from build123d import *

# Parameters (mm, degrees)
SKETCH1_R                                   = 16
BOSS_EXTRUDE1_DEPTH                         = 7.5
SKETCH2_W                                   = 15
SKETCH2_H                                   = 17
BOSS_EXTRUDE2_DEPTH                         = 20
SKETCH3_W                                   = 70
SKETCH3_H                                   = 50
SKETCH3_R                                   = 12.5
SKETCH3_R_2                                 = 1.75
BOSS_EXTRUDE4_DEPTH                         = 15
CHAMFER1_SIZE                               = 1
CUT_EXTRUDE1_REACH                          = 72.373
SKETCH4_R                                   = 3.5
CBORE_FOR_M3_CHEESE_HEAD_SCREW3_D           = 3.4
CBORE_FOR_M3_CHEESE_HEAD_SCREW3_CBORE_D     = 6.5
CBORE_FOR_M3_CHEESE_HEAD_SCREW3_CBORE_DEPTH = 2
BOSS_EXTRUDE5_START                         = -17
BOSS_EXTRUDE5_DEPTH                         = 17
CBORE_FOR_M6_HEX_HEAD_BOLT1_AT_2_COUNT      = 2
CBORE_FOR_M6_HEX_HEAD_BOLT1_AT_2_PITCH      = 18
CBORE_FOR_M6_HEX_HEAD_BOLT1_AT_3_COUNT      = 2
CBORE_FOR_M6_HEX_HEAD_BOLT1_AT_3_PITCH      = 68.410525506
CBORE_FOR_M6_HEX_HEAD_BOLT1_AT_4_COUNT      = 2
CBORE_FOR_M6_HEX_HEAD_BOLT1_AT_4_PITCH      = 66


# Read off the part's stored shape, not the designer's step: Boss-Extrude5
with BuildPart() as part:
    # Sketch1 → Boss-Extrude1 (new, symmetric)
    with BuildSketch(Plane.XY):
        Polygon((-25, -20.805513048), (-40, -20.805513048), (-40, -3.805513048), (-25, -3.805513048), (-25, 29.194486952), (25, 29.194486952), (25, -3.805513048), (40, -3.805513048), (40, -20.805513048), (25, -20.805513048), align=None)
        with Locations((0, 4.194486952)):
            Circle(SKETCH1_R, mode=Mode.SUBTRACT)
    extrude(amount=BOSS_EXTRUDE1_DEPTH, both=True)

    # Sketch2 → Boss-Extrude2 (add)
    with BuildSketch(Plane(origin=(0, 0, -7.5), x_dir=(-1, 0, 0), z_dir=(0, 0, -1))):
        with Locations((32.5, -12.305513048)):
            Rectangle(SKETCH2_W, SKETCH2_H)
        with Locations((-32.5, -12.305513048)):
            Rectangle(SKETCH2_W, SKETCH2_H)
    extrude(amount=BOSS_EXTRUDE2_DEPTH)

    # Sketch3 → Boss-Extrude4 (add)
    with BuildSketch(Plane(origin=(0, 0, -27.5), x_dir=(-1, 0, 0), z_dir=(0, 0, -1))):
        with Locations((-5, 4.194486952)):
            Rectangle(SKETCH3_W, SKETCH3_H)
        with Locations((0, 4.194486952)):
            Circle(SKETCH3_R, mode=Mode.SUBTRACT)
        with Locations((15.5, 19.694486952)):
            Circle(SKETCH3_R_2, mode=Mode.SUBTRACT)
        with Locations((-15.5, 19.694486952)):
            Circle(SKETCH3_R_2, mode=Mode.SUBTRACT)
        with Locations((15.5, -11.305513048)):
            Circle(SKETCH3_R_2, mode=Mode.SUBTRACT)
        with Locations((-15.5, -11.305513048)):
            Circle(SKETCH3_R_2, mode=Mode.SUBTRACT)
    extrude(amount=BOSS_EXTRUDE4_DEPTH)

    # Chamfer1
    chamfer1_edges = [part.edges().sort_by_distance(p)[0] for p in [
        (0, 29.194486952, -7.5),
        (-25, 29.194486952, 0),
        (25, 29.194486952, 0),
        (40, -3.805513048, -10),
        (40, -12.305513048, 7.5),
        (32.5, -3.805513048, 7.5),
        (25, 12.694486952, 7.5),
        (-25, -3.805513048, -17.5),
        (0, 29.194486952, 7.5),
        (25, -3.805513048, -17.5),
        (-25, 12.694486952, 7.5),
        (40, 12.694486952, -27.5),
        (5, 29.194486952, -27.5),
        (40, 4.194486952, -42.5),
        (40, 29.194486952, -35),
        (-30, 12.694486952, -27.5),
        (5, 29.194486952, -42.5),
        (-30, 29.194486952, -35),
        (-30, 4.194486952, -42.5),
    ]]
    chamfer(chamfer1_edges, length=CHAMFER1_SIZE)

    # Sketch4 → Cut-Extrude1 (cut, up to next)
    with BuildSketch(Plane.XY.offset(7.5), mode=Mode.PRIVATE) as cut_extrude1_sk1:
        with Locations((-15.5, 19.694486952)):
            Circle(SKETCH4_R)
    cut_extrude1_tool1 = extrude(cut_extrude1_sk1.sketch, amount=-CUT_EXTRUDE1_REACH, mode=Mode.PRIVATE) & part.part
    # Sketch4 → Cut-Extrude1 (cut, up to next)
    with BuildSketch(Plane.XY.offset(7.5), mode=Mode.PRIVATE) as cut_extrude1_sk2:
        with Locations((-15.5, -11.305513048)):
            Circle(SKETCH4_R)
    cut_extrude1_tool2 = extrude(cut_extrude1_sk2.sketch, amount=-CUT_EXTRUDE1_REACH, mode=Mode.PRIVATE) & part.part
    # Sketch4 → Cut-Extrude1 (cut, up to next)
    with BuildSketch(Plane.XY.offset(7.5), mode=Mode.PRIVATE) as cut_extrude1_sk3:
        with Locations((15.5, -11.305513048)):
            Circle(SKETCH4_R)
    cut_extrude1_tool3 = extrude(cut_extrude1_sk3.sketch, amount=-CUT_EXTRUDE1_REACH, mode=Mode.PRIVATE) & part.part
    # Sketch4 → Cut-Extrude1 (cut, up to next)
    with BuildSketch(Plane.XY.offset(7.5), mode=Mode.PRIVATE) as cut_extrude1_sk4:
        with Locations((15.5, 19.694486952)):
            Circle(SKETCH4_R)
    cut_extrude1_tool4 = extrude(cut_extrude1_sk4.sketch, amount=-CUT_EXTRUDE1_REACH, mode=Mode.PRIVATE) & part.part
    add(cut_extrude1_tool1.solids().sort_by_distance((-15.5, 19.694487, 7.5))[0], mode=Mode.SUBTRACT)
    add(cut_extrude1_tool2.solids().sort_by_distance((-15.5, -11.305513, 7.5))[0], mode=Mode.SUBTRACT)
    add(cut_extrude1_tool3.solids().sort_by_distance((15.5, -11.305513, 7.5))[0], mode=Mode.SUBTRACT)
    add(cut_extrude1_tool4.solids().sort_by_distance((15.5, 19.694487, 7.5))[0], mode=Mode.SUBTRACT)

    # CBORE for M3 Cheese Head Screw3 (through all)
    with Locations(Plane(origin=(-15.5, 19.694486952, -27.5), x_dir=(1, 0, 0), z_dir=(0, 0, 1))):
        with Locations((0, 0), (31, 0), (0, -31), (31, -31)):
            CounterBoreHole(CBORE_FOR_M3_CHEESE_HEAD_SCREW3_D / 2, CBORE_FOR_M3_CHEESE_HEAD_SCREW3_CBORE_D / 2, CBORE_FOR_M3_CHEESE_HEAD_SCREW3_CBORE_DEPTH)

    # Boss-Extrude5 outline → Boss-Extrude5 (add)
    with BuildSketch(Plane(origin=(0, -3.805513048, 0), x_dir=(1, 0, 0), z_dir=(0, 1, 0)).offset(BOSS_EXTRUDE5_START)):
        with BuildLine():
            Line((-40, -3.741657387), (-40, 27.5))
            Line((-40, 27.5), (-30, 27.5))
            Line((-30, 27.5), (-30, 32.133249581))
            ThreePointArc((-30, 32.133249581), (-37.372983346, 31.922616289), (-41, 25.5))
            Line((-41, 25.5), (-41, 0))
            ThreePointArc((-41, 0), (-40.745688373, -1.936491673), (-40, -3.741657387))
        make_face()
        with BuildLine():
            Line((41, 0), (41, 25.5))
            ThreePointArc((41, 25.5), (28.196699141, 30.803300859), (33.5, 18))
            Line((33.5, 18), (33.5, 7.5))
            ThreePointArc((33.5, 7.5), (26.254311627, 1.936491673), (29.758342613, -6.5))
            ThreePointArc((29.758342613, -6.5), (33.5, -7.5), (37.241657387, -6.5))
            ThreePointArc((37.241657387, -6.5), (39.992781777, -3.754168989), (41, 0))
        make_face()
    extrude(amount=BOSS_EXTRUDE5_DEPTH)

    # Sketch9 → CBORE for M6 Hex Head Bolt1 (revolve, cut)
    with BuildSketch(Plane(origin=(-33, -3.805513048, -3), x_dir=(0, 0, 1), z_dir=(1, 0, 0))):
        Polygon((0, 0), (0, 17), (3.3, 17), (3.3, 4.38), (7.275, 4.38), (7.275, 0), align=None)
    cbore_for_m6_hex_head_bolt1 = revolve(axis=Axis((-33, 2.544486952, -3), (0, -1, 0)), mode=Mode.SUBTRACT)

    # CBORE for M6 Hex Head Bolt1 at 2: CBORE for M6 Hex Head Bolt1 ×2
    with Locations(*[(0, 0, -i * CBORE_FOR_M6_HEX_HEAD_BOLT1_AT_2_PITCH) for i in range(1, CBORE_FOR_M6_HEX_HEAD_BOLT1_AT_2_COUNT)]):
        add(cbore_for_m6_hex_head_bolt1, mode=Mode.SUBTRACT)

    # CBORE for M6 Hex Head Bolt1 at 3: CBORE for M6 Hex Head Bolt1 ×2
    with Locations(*[Vector(0.9647638212377322, 0, -0.26311740579210874) * (i * CBORE_FOR_M6_HEX_HEAD_BOLT1_AT_3_PITCH) for i in range(1, CBORE_FOR_M6_HEX_HEAD_BOLT1_AT_3_COUNT)]):
        add(cbore_for_m6_hex_head_bolt1, mode=Mode.SUBTRACT)

    # CBORE for M6 Hex Head Bolt1 at 4: CBORE for M6 Hex Head Bolt1 ×2
    with Locations(*[(i * CBORE_FOR_M6_HEX_HEAD_BOLT1_AT_4_PITCH, 0, 0) for i in range(1, CBORE_FOR_M6_HEX_HEAD_BOLT1_AT_4_COUNT)]):
        add(cbore_for_m6_hex_head_bolt1, mode=Mode.SUBTRACT)


solid = part.part
Source: CAD feature listing. Evaluate the final solid. Frame: model axes, mm. A direction names the side the tool comes from. Round coordinates to 2 decimals unless told otherwise and drop trailing zeros. Loops run counter-clockwise (first coordinate to the right, second up) from the corner with the lowest first, then second, coordinate; pieces in that order, holes last. Notation, with made-up numbers: (19, 37) -> (31, 37) arc R16 cw to (31, 47) -> close; hole circle Ø1 at (88, -37.5). An arc over 180 degrees is marked (long way). Answer as a JSON object with one key per item and string values. Group by question number.
Q1. Ray query, line 1 (X direction, y = 21, z = -3.5); line 2 (X direction, y = -16.25, z = -3); line 3 (Z direction, x = -10.5, y = 23). Return the intervals inside material, ascending. Write a range as from..to.
Q2. Section query A-A (x = 3.5). Output: boundary loops of the cut face in (y, z), plus the area to 3 significant figures.
Q3. Contact query for flat-ended pins moving along their axis: P1, Ø2, axis at y = 22, z = -1.5, coming from the +X side; P2, Ø4, axis at x = 28, z = -26, coming from the +Y side; P3, Ø6.5, axis at y = -7.5, z = -32, coming from the +X side; P4, Ø3, axis at y = 1, z = -25.5, coming from the +X side. Output: stop coordinate, or through.
Q4. Mould query, pull axis X, two halves, no side actions, for faces 4 (the cylindrical face through (40.753, -12.425, -27.41)), 5 (the flat face through (-25, -13, -17)), 6 (the cylindrical face through (-40.753, -12.425, 1.91)). Classes: pulls with the +X half, pulls with the -X half, needs draft (parallel to the pull), parting line crosses it, or undercut.
Q5. Section query B-B (z = -1). State how many separate pieces and enclosed holes the cut face has, plus the area to 3 significant figures.
Q6. Section query C-C (y = -1.5). Output: boundary loops of the cut face in (x, z), plus the area to 3 significant figures.
Q7. Access query for faces 1 (the cylindrical face through (17.12, 16.59, 0.11)), 2 (the cylindrical face through (13.883, -11.976, -35.909)), 3 (the cylindrical face through (-40.213, -5.965, -21.947)). Directions: +Z, -Z, +X, -X, +Y, -Y. A direction counts if a zero-diameter tool reaches every point of the face in a straight line with its end or side. Return the directions, or none.
Q8. Section query D-D (z = -21). Output: boundary loops of the cut face in (x, y) (3 decimals).
Completed:
{
 "1": {"line 1": "-25..-18.75, -12.25..12.25, 18.75..25", "line 2": "-41..-36.3, -29.7..29.7, 36.3..41", "line 3": "-42.5..-27.5, -7.5..7.5"},
 "2": {"outline": "(-20.81, -42.5) -> (-7.81, -42.5) -> (-7.81, -27.5) -> (-20.81, -27.5) -> close; (-20.81, -7.5) -> (-11.42, -7.5) -> (-11.42, 7.5) -> (-20.81, 7.5) -> close; (16.19, -42.5) -> (28.19, -42.5) -> (29.19, -41.5) -> (29.19, -28.5) -> (28.19, -27.5) -> (16.19, -27.5) -> close; (19.81, -7.5) -> (28.19, -7.5) -> (29.19, -6.5) -> (29.19, 6.5) -> (28.19, 7.5) -> (19.81, 7.5) -> close", "area": "670 mm²"},
 "3": {"P1": "x = 25", "P2": "y = 28.69", "P3": "x = 40.26", "P4": "through"},
 "4": {"face 4": "pulls with the +X half", "face 5": "undercut", "face 6": "pulls with the -X half"},
 "5": {"separate pieces": "3", "enclosed holes": "5", "area": "1,830 mm²"},
 "6": {"outline": "(-30, -41.5) -> (-29, -42.5) -> (-11.13, -42.5) -> (-11.13, -27.5) -> (-29, -27.5) -> (-30, -28.5) -> close; (-25, -7.5) -> (-14.95, -7.5) -> (-14.95, 7.5) -> (-24, 7.5) -> (-25, 6.5) -> close; (11.13, -42.5) -> (39, -42.5) -> (40, -41.5) -> (40, -28.5) -> (39, -27.5) -> (11.13, -27.5) -> close; (14.95, -7.5) -> (25, -7.5) -> (25, 6.5) -> (24, 7.5) -> (14.95, 7.5) -> close", "area": "1,010 mm²"},
 "7": {"face 1": "+Z", "face 2": "+Z, -Z", "face 3": "+Y"},
 "8": {"outline": "(-41, -20.806) -> (-36.3, -20.806) -> (-36.3, -8.186) -> (-40.275, -8.186) -> (-40.275, -3.806) -> (-41, -3.806) -> close; (-29.7, -20.806) -> (-25, -20.806) -> (-25, -4.806) -> (-25.725, -4.081) -> (-25.725, -8.186) -> (-29.7, -8.186) -> close; (25, -20.806) -> (29.7, -20.806) -> (29.7, -8.186) -> (25.725, -8.186) -> (25.725, -4.081) -> (25, -4.806) -> close; (36.3, -20.806) -> (41, -20.806) -> (41, -3.806) -> (40.275, -3.806) -> (40.275, -8.186) -> (36.3, -8.186) -> close"}
}
